Source: three-view drawing plus pictorial views. Frame: mm from the lowest corner of the part. Round coordinates to 2 decimals unless told otherwise and drop trailing zeros. Loops run counter-clockwise (first coordinate to the right, second up) from the corner with the lowest first, then second, coordinate; pieces in that order, holes last. Notation, with made-up numbers: M 48,44 L 79,44 A31 cw 79,82 Z; hole C -25.5,-29 d4. An arc over 180 degrees is marked long. Write each question's results on one line, items separated by ' | '.
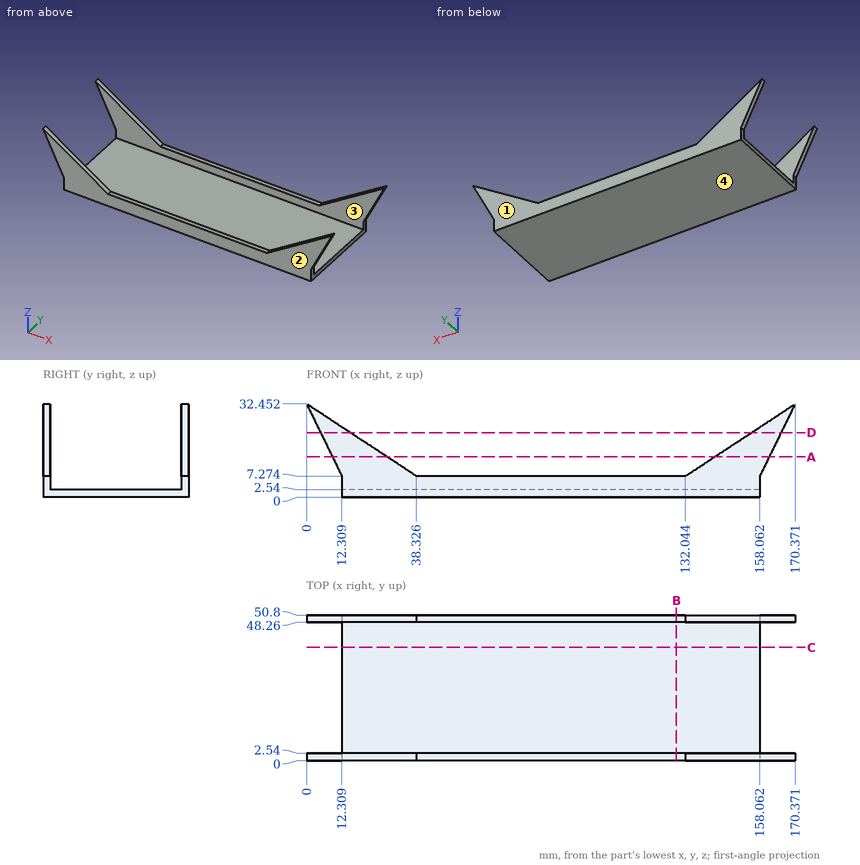
1. Ray query, probe 1 along Y at (x, z) = (60, 7); probe 2 along Z at (x, y) = (62.5, 9.5); probe 3 along Z at (x, y) = (130, 48.5). Return the intervals inside material, ascending.
Answer key:
probe 1: y = 0 to 2.54, 48.26 to 50.8 | probe 2: z = 0 to 2.54 | probe 3: z = 0 to 7.27
2. Section C-C (y = 39.5). Output: boundary loops of the cut face in (x, z), then the cut area to 3 significant figures.
Answer key:
outline: M 12.31,0 L 158.06,0 L 158.06,2.54 L 12.31,2.54 Z | area: 370 mm²
3. Section B-B (x = 129). Output: boundary loops of the cut face in (y, z).
Answer key:
outline: M 0,0 L 50.8,0 L 50.8,7.27 L 48.26,7.27 L 48.26,2.54 L 2.54,2.54 L 2.54,7.27 L 0,7.27 Z
4. Pin query (flat end, axial travel): P1, Ø6, axis at y = 21.5, z = 2, coming from the +X side; P2, Ø1.3, axis at x = 108, y = 0.5, coming from the +Z side; P3, Ø12, axis at y = 43.5, z = 17, coming from the +X side. Return the tip coordinate at first contact, or that it passes through.
Answer key:
P1: stops at x = 158.06 | P2: stops at z = 7.27 | P3: stops at x = 164.6
5. Section A-A (z = 14). Output: boundary loops of the cut face in (x, y).
Answer key:
outline: M 9.02,0 L 28.09,0 L 28.09,2.54 L 9.02,2.54 Z; M 9.02,48.26 L 28.09,48.26 L 28.09,50.8 L 9.02,50.8 Z; M 142.28,0 L 161.35,0 L 161.35,2.54 L 142.28,2.54 Z; M 142.28,48.26 L 161.35,48.26 L 161.35,50.8 L 142.28,50.8 Z
6. Draft query along Y for the marked faces 1, 2, 3 and 4. Return one class per face: pulls with the +Y half, pulls with the -Y half, needs draft (parallel to the pull), parting line crosses it, or undercut.
Answer key:
face 1: pulls with the +Y half | face 2: pulls with the -Y half | face 3: undercut | face 4: needs draft
7. Section D-D (z = 22.5). Output: boundary loops of the cut face in (x, y) (1 decimal).
Answer key:
outline: M 4.9,0 L 15.1,0 L 15.1,2.5 L 4.9,2.5 Z; M 4.9,48.3 L 15.1,48.3 L 15.1,50.8 L 4.9,50.8 Z; M 155.2,0 L 165.5,0 L 165.5,2.5 L 155.2,2.5 Z; M 155.2,48.3 L 165.5,48.3 L 165.5,50.8 L 155.2,50.8 Z
